Part model, mm, in its own coordinate system. Coordinates: 2 decimals unless noted, no trailing zeros. Loops run counter-clockwise (first coordinate to the right, second up) from the corner with the lowest first, then second, coordinate; pieces in that order, holes last. Notation, with made-up numbers: (50.25, 21.25) - (88.25, 21.25) arc R11 ccw to (88.25, 28.25) - close; hole circle Ø1 at (-27.75, 7.5). An arc over 180 degrees is marked (long way). Use a Markdown table: item, result. Add a question column.
1. Band-saw the part on B-B, the plane x = 7.5. Give the cut face in (y, z).
2. Drop flat-ended pins along their axis: pin 1 (1 mm diameter, centred on x = 47, y = 8.5, fed in from -Z); pin 2 (4 mm diameter, centred on x = 52.37, y = 12.63, fed in from +Z). Give the stop position or say it passes through.
3. Band-saw the part on A-A, the plane x = 40. Give the cut face in (y, z), plus the area to 3 significant figures.
4. Band-saw the part on D-D, the plane y = 33.5. Give the cut face in (x, z).
5. Wall check: probe 1 along Y at (x, z) = (72.5, 0.75); probe 2 along X at (y, z) = (10, 1.9); probe 3 along X at (y, z) = (13.5, 0.65). Give the ranges that are in metal, low to high. Write a range as [from, to].
6. Band-saw the part on C-C, the plane z = 1.35. Count the separate pieces of the cut face and the enclosed holes in it, plus the area to 3 significant figures.
Autodesk Inventor part; units mm, degrees
ref_plane "YZ Plane" through (0, 0, 0) normal (1, 0, 0) x (0, 1, 0)
ref_plane "XZ Plane" through (0, 0, 0) normal (0, 1, 0) x (-1, 0, 0)
ref_plane "XY Plane" through (0, 0, 0) normal (0, 0, 1) x (1, 0, 0)
sketch "スケッチ1" plane through (0, 0, 0) normal (0, 0, 1) x (1, 0, 0)
  line L0 (0, 0) -> (80, 0)
  line L1 (80, 0) -> (80, 50)
  line L2 (80, 50) -> (0, 50)
  line L3 (0, 50) -> (0, 0)
  dimension "d0" = 80
  dimension "d1" = 50
extrude "押し出し1" add sketch "スケッチ1" along normal blind 3
sketch "スケッチ2" plane through (0, 0, 3) normal (0, 0, 1) x (1, 0, 0)
  circle A0 centre (40, 25) radius 13
  line L0 (80, 50) -> (0, 50)
  line L1 (0, 50) -> (0, 0)
  dimension "d4" = 26
  dimension "d5" = 25
  dimension "d6" = 40
extrude "押し出し2" cut sketch "スケッチ2" against normal blind 3
sketch "スケッチ3" plane through (0, 0, 3) normal (0, 0, 1) x (1, 0, 0)
  circle A0 centre (40, 25) radius 13
  circle A1 centre (40, 25) radius 17.5 construction
  line L0 (40, 25) -> (57.5, 25)
  line L1 (40, 25) -> (53, 36.7154) construction
  line L2 (53, 36.7154) -> (19.5714, 6.5901) construction
  line L3 (40, 25) -> (52.3744, 12.6256)
  line L4 (40, 25) -> (57.5, 25) construction
  line L5 (52.3744, 12.6256) -> (27.6256, 37.3744) construction
  circle A2 centre (53, 36.7154) radius 2.1
  circle A3 centre (27.6256, 37.3744) radius 2.1
  circle A4 centre (27, 13.2846) radius 2.1
  circle A5 centre (52.3744, 12.6256) radius 2.1
  point P0 (0, 0)
  dimension "d9" = 35
  dimension "d10" = 17.5
  dimension "d11" = 45
  dimension "d12" = 45
  dimension "d13" = 4.2
  dimension "d14" = 4.2
  dimension "d15" = 4.2
  dimension "d16" = 4.2
hole "穴1" at (27.6256, 37.3744, 3) at (53, 36.7154, 3) at (27, 13.2846, 3) at (52.3744, 12.6256, 3) direction (0, 0, -1) diameter 4.2 end through all
sketch "スケッチ4" plane through (0, 0, 3) normal (0, 0, 1) x (1, 0, 0)
  line L0 (80, 50) -> (0, 50)
  line L1 (15, 50) -> (15, 0) construction
  line L2 (0, 0) -> (80, 0)
  line L3 (65, 50) -> (65, 0) construction
  line L4 (0, 50) -> (0, 0)
  line L5 (80, 0) -> (80, 50)
  circle A0 centre (7.5, 40) radius 1.6
  circle A1 centre (7.5, 25) radius 1.6
  circle A2 centre (7.5, 10) radius 1.6
  circle A3 centre (72.5, 40) radius 1.6
  circle A4 centre (72.5, 25) radius 1.6
  circle A5 centre (72.5, 10) radius 1.6
  point P0 (40, 0)
  dimension "d24" = 15
  dimension "d25" = 15
  dimension "d26" = 3.2
  dimension "d27" = 7.5
  dimension "d28" = 10
  dimension "d29" = 3.2
  dimension "d30" = 3.2
  dimension "d31" = 25
  dimension "d32" = 10
  dimension "d33" = 7.5
  dimension "d34" = 7.5
hole "穴2" at (7.5, 40, 3) at (7.5, 25, 3) at (7.5, 10, 3) at (72.5, 40, 3) at (72.5, 25, 3) at (72.5, 10, 3) direction (0, 0, -1) diameter 3.2 end through all
fillet "フィレット1" radius 3 4 edges at (0, 50, 1.5) (80, 50, 1.5) (80, 0, 1.5) (0, 0, 1.5)
properties part number "射出_モーター固定1" material "アルミニウム 6061"
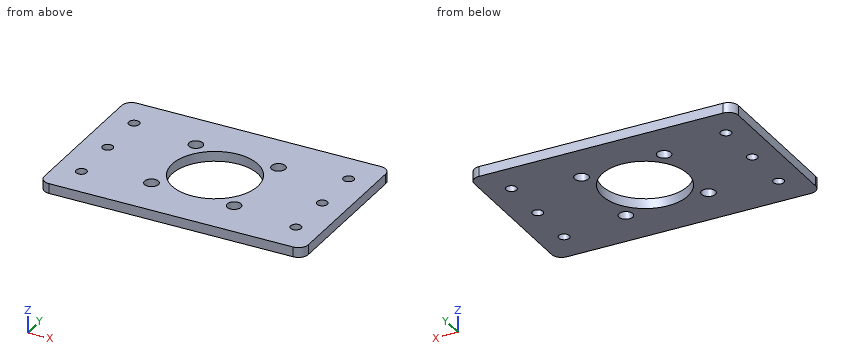
Geometry check:
| question | item | result |
|---|---|---|
| 1 | outline | (0, 0) - (8.4, 0) - (8.4, 3) - (0, 3) - close; (11.6, 0) - (23.4, 0) - (23.4, 3) - (11.6, 3) - close; (26.6, 0) - (38.4, 0) - (38.4, 3) - (26.6, 3) - close; (41.6, 0) - (50, 0) - (50, 3) - (41.6, 3) - close |
| 2 | pin 1 | stops at z = 0 |
| 2 | pin 2 | passes through |
| 3 | outline | (0, 0) - (12, 0) - (12, 3) - (0, 3) - close; (38, 0) - (50, 0) - (50, 3) - (38, 3) - close |
| 3 | area | 72.0 mm^2 |
| 4 | outline | (0, 0) - (30.16, 0) - (30.16, 3) - (0, 3) - close; (49.84, 0) - (80, 0) - (80, 3) - (49.84, 3) - close |
| 5 | probe 1 | y = [0, 8.4], [11.6, 23.4], [26.6, 38.4], [41.6, 50] |
| 5 | probe 2 | x = [0, 5.9], [9.1, 70.9], [74.1, 80] |
| 5 | probe 3 | x = [0, 24.91], [29.09, 33.94], [46.06, 50.47], [54.28, 80] |
| 6 | separate pieces | 1 |
| 6 | enclosed holes | 11 |
| 6 | area | 3,360 mm^2 |
